from build123d import *

# Parameters (mm, degrees)
F0_W     = 209.55
F0_H     = 76.2
F1_DEPTH = 76.2
F2_W     = 209.55
F2_H     = 38.1
F3_DEPTH = 38.1
F4_R     = 11.1125
F4_R_2   = 11.325083
F5_DEPTH = 19.05
F6_R     = 11.1125
F7_DEPTH = 19.05


with BuildPart() as f1:
    # F0 (on Front) → F1 (new body)
    with BuildSketch(Plane.XZ):
        with Locations((30.458469, 38.1)):
            Rectangle(F0_W, F0_H)
    extrude(amount=F1_DEPTH)

    # F2 (on face) → F3 (cut)
    with BuildSketch(Plane.XZ.offset(76.2)):
        with Locations((30.458469, 19.05)):
            Rectangle(F2_W, F2_H)
    extrude(amount=-F3_DEPTH, mode=Mode.SUBTRACT)

    # F4 (on face) → F5 (cut)
    with BuildSketch(Plane.XZ.offset(38.1)):
        with Locations((-56.854031, 19.05)):
            Circle(F4_R)
        with Locations((-28.279031, 19.05)):
            Circle(F4_R)
        with Locations((0.295969, 19.05)):
            Circle(F4_R)
        with Locations((57.445969, 19.05)):
            Circle(F4_R)
        with Locations((86.020969, 19.05)):
            Circle(F4_R)
        with Locations((114.595969, 19.05)):
            Circle(F4_R_2)
        with Locations((28.870969, 19.05)):
            Circle(F4_R)
    extrude(amount=-F5_DEPTH, mode=Mode.SUBTRACT)

    # F6 (on face) → F7 (cut)
    with BuildSketch(Plane.XZ.offset(76.2)):
        with Locations((-42.566531, 57.15)):
            Circle(F6_R)
        with Locations((-13.991531, 57.15)):
            Circle(F6_R)
        with Locations((14.583469, 57.15)):
            Circle(F6_R)
        with Locations((43.158469, 57.15)):
            Circle(F6_R)
        with Locations((71.733469, 57.15)):
            Circle(F6_R)
        with Locations((100.308469, 57.15)):
            Circle(F6_R)
    extrude(amount=-F7_DEPTH, mode=Mode.SUBTRACT)


solid = f1.part
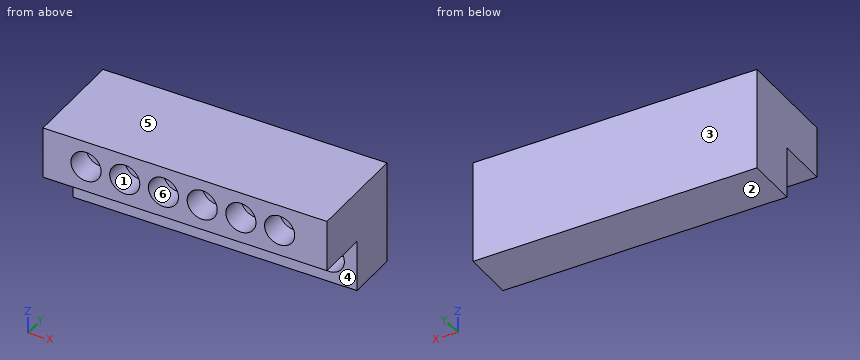
The model under review builds one solid part; all positions refer to its coordinate system, in mm. Face numbers are marked on the shaded views. A direction names the side the tool comes from. Round coordinates to 2 decimals unless told otherwise and drop trailing zeros. Order: outer loops, then holes, each group sorted by start corner. A loop starts at its lowest first (then second) coordinate and runs counter-clockwise, first axis right, second up. Notation, with made-up numbers: (60, 66.25) -> (80, 66.25) arc R18 ccw to (80, 73.25) -> close; hole circle Ø7 at (66, -34.5). An arc over 180 degrees is marked (long way). Return JSON: item names as keys, results as strings.
1. For the marked faces 4, 5 and 6, list the 3-axis set-ups (+Z, -Z, +X, -X, +Y, -Y) from which the entire face can be reached by the end or side of a thin tool; tool diameter is ignored.
Answer block:
{"face 4": "-Z, +X, -X, -Y", "face 5": "+Z, +X, -X, +Y, -Y", "face 6": "-Y"}
2. For L1, parallel to Z at x = -28.5, y = -36; L2, parallel to Y at x = 36, z = 30; L3, parallel to Z at x = 44.5, y = -44, list the stretches that pass through material, from the lowest coordinate up. Write a range as [from, to].
Answer block:
{"L1": "z = [0, 7.94], [30.16, 76.2]", "L2": "y = [-38.1, 0]", "L3": "z = [38.1, 76.2]"}
3. Insertion check: P1, Ø10, axis at x = 55.5, y = -45, coming from the -Z side; P2, Ø11, axis at x = 88, z = 16.5, coming from the -Y side; P3, Ø6.5, axis at x = 45.5, z = 54.5, coming from the -Y side. Each pin has a flat end and moves straight along its axis. Give the tip position at first contact, or say it passes through.
Answer block:
{"P1": "stops at z = 38.1", "P2": "stops at y = -19.05", "P3": "stops at y = -57.15"}
4. Take a section at A-A (y = -67). State how many separate pieces and enclosed holes the cut face has, then the cut area to 3 significant figures.
Answer block:
{"separate pieces": "1", "enclosed holes": "6", "area": "5,660 mm²"}
5. Take a section at B-B (z = 57.15). Write out the cut boundary in (x, y).
Answer block:
{"outline": "(-74.32, -76.2) -> (-53.68, -76.2) -> (-53.68, -57.15) -> (-31.45, -57.15) -> (-31.45, -76.2) -> (-25.1, -76.2) -> (-25.1, -57.15) -> (-2.88, -57.15) -> (-2.88, -76.2) -> (3.47, -76.2) -> (3.47, -57.15) -> (25.7, -57.15) -> (25.7, -76.2) -> (32.05, -76.2) -> (32.05, -57.15) -> (54.27, -57.15) -> (54.27, -76.2) -> (60.62, -76.2) -> (60.62, -57.15) -> (82.85, -57.15) -> (82.85, -76.2) -> (89.2, -76.2) -> (89.2, -57.15) -> (111.42, -57.15) -> (111.42, -76.2) -> (135.23, -76.2) -> (135.23, 0) -> (-74.32, 0) -> close"}
6. Take a section at C-C (y = -45.5). Write out the cut boundary in (x, z), then the cut area to 3 significant figures.
Answer block:
{"outline": "(-74.32, 38.1) -> (135.23, 38.1) -> (135.23, 76.2) -> (-74.32, 76.2) -> close", "area": "7,980 mm²"}
7. The part is to be moulded in two halves that separate along Z. For the marked faces 1, 2 and 3, say which applies: +Z half, -Z half, draft (parallel to the pull), parting line (faces both ways), or undercut.
Answer block:
{"face 1": "undercut", "face 2": "-Z half", "face 3": "draft"}
